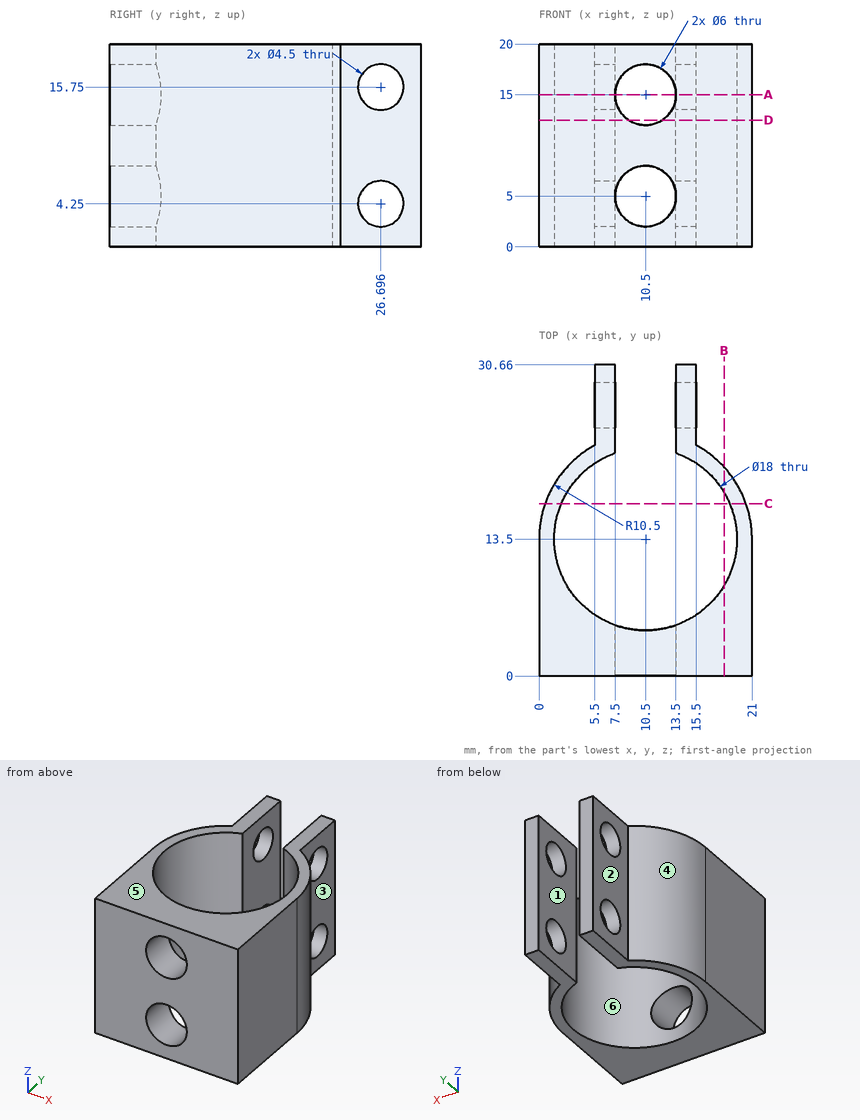
Verification items for this drawing (mm, ordinates from the low corner). A direction names the side the tool comes from. Give positions to 0.01 mm unless a question says otherwise; leave off trailing zeros. Write each loop counter-clockwise with the first axis right and the second up, starting at its lowest first coordinate (ties: lowest second). Pieces come first, ordered by that corner, then holes. Notation, with made-up numbers: M -28,65 L 6,65 A25 ccw 6,84 Z; hole C -2,75 d11. An arc over 180 degrees is marked long. Use one line per item in the form item = value.
(1) Section check A-A on z = 15. Record the boundary of the cut face in (x, y) (1 decimal).
Answer block:
outline = M 0,0 L 7.5,0 L 7.5,5 A9 cw 7.5,22 L 7.5,24.6 L 5.5,24.6 L 5.5,22.7 A10.5 ccw 0,13.5 Z; M 5.5,28.8 L 7.5,28.8 L 7.5,30.7 L 5.5,30.7 Z; M 13.5,0 L 21,0 L 21,13.5 A10.5 ccw 15.5,22.7 L 15.5,24.6 L 13.5,24.6 L 13.5,22 A9 cw 13.5,5 Z; M 13.5,28.8 L 15.5,28.8 L 15.5,30.7 L 13.5,30.7 Z
(2) Depth check by flat-ended pin: P1, Ø8.5, axis at y = 25.5, z = 14, coming from the +X side (1 decimal); P2, Ø9.5, axis at y = 27, z = 8, coming from the -X side (1 decimal); P3, Ø4, axis at y = 26.7, z = 15.75, coming from the -X side; P4, Ø1, axis at x = 18, z = 12, coming from the +Y side (1 decimal). Enter the tip coordinate at first touch or a pass-through.
Answer block:
P1 = 17.6
P2 = 4.7
P3 = through
P4 = 21.3
(3) Section check B-B on x = 18.25. Record the boundary of the cut face in (y, z) (1 decimal), plus the area to 3 significant figures.
Answer block:
outline = M 0,0 L 8.9,0 L 8.9,20 L 0,20 Z; M 18.1,0 L 20.6,0 L 20.6,20 L 18.1,20 Z
area = 229 mm2
(4) Section check D-D on z = 12.5. Record the boundary of the cut face in (x, y) (1 decimal), plus the area to 3 significant figures.
Answer block:
outline = M 0,0 L 8.8,0 L 8.8,4.7 A9 cw 7.5,22 L 7.5,30.7 L 5.5,30.7 L 5.5,22.7 A10.5 ccw 0,13.5 Z; M 12.2,0 L 21,0 L 21,13.5 A10.5 ccw 15.5,22.7 L 15.5,30.7 L 13.5,30.7 L 13.5,22 A9 cw 12.2,4.7 Z
area = 208 mm2
(5) Tool access check on the marked faces 1, 2 and 3. Record the directions out of +Z, -Z, +X, -X, +Y, -Y that give a thin tool (end or side, any length) a straight path to the whole face; none if there is none.
Answer block:
face_1 = +Z, -Z, +Y
face_2 = +Z, -Z, -X, +Y
face_3 = +Z, -Z, +X, +Y
(6) Draft check along X on the marked faces 4, 5 and 6. Enter one of: pulls with the +X half, pulls with the -X half, needs draft (parallel to the pull), parting line crosses it, or undercut.
Answer block:
face_4 = pulls with the -X half
face_5 = needs draft
face_6 = undercut
(7) Material ranges on line 1 along X through (y, z) = (23.5, 16.25); line 2 along Z through (x, y) = (10.5, 3.05); line 3 along Y through (x, z) = (14.75, 17.75) (1 decimal), recorded low to high.
Answer block:
line_1 = 5.5 to 7.5, 13.5 to 15.5
line_2 = 0 to 2, 8 to 12, 18 to 20
line_3 = 0 to 5.6, 21.4 to 25.7, 27.7 to 30.7
(8) Section check C-C on y = 17. Record the boundary of the cut face in (x, z).
Answer block:
outline = M 0.6,0 L 2.21,0 L 2.21,20 L 0.6,20 Z; M 18.79,0 L 20.4,0 L 20.4,20 L 18.79,20 Z
